```python
from build123d import *

# Parameters (mm, degrees)
SKETCH1_W           = 22
SKETCH1_H           = 22
BOSS_EXTRUDE1_DEPTH = 63.5
CUT_EXTRUDE1_DEPTH  = 71.712445864
SKETCH3_W           = 3
SKETCH3_H           = 7
CUT_EXTRUDE2_DEPTH  = 71.712445864
BOSS_EXTRUDE2_REACH = 68.259
SKETCH4_W           = 7
SKETCH4_H           = 2
FILLET1_R           = 2
CHAMFER1_SIZE       = 3


with BuildPart() as part:
    # Sketch1 → Boss-Extrude1 (new body)
    with BuildSketch(Plane.XY):
        with Locations((11, 11)):
            Rectangle(SKETCH1_W, SKETCH1_H)
    extrude(amount=-BOSS_EXTRUDE1_DEPTH)

    # Sketch2 → Cut-Extrude1 (cut, through all)
    with BuildSketch(Plane(origin=(22, 0, 0), x_dir=(0, 0, -1), z_dir=(1, 0, 0))):
        Polygon((5, 22), (5, 15), (22.833333333, 15), (22.833333333, 17), (40.666666667, 17), (40.666666667, 15), (58.5, 15), (58.5, 22), align=None)
        Polygon((22.833333333, 7), (22.833333333, 5), (40.666666667, 5), (40.666666667, 7), (58.5, 7), (58.5, 0), (5, 0), (5, 7), align=None)
    extrude(amount=-CUT_EXTRUDE1_DEPTH, mode=Mode.SUBTRACT)

    # Sketch3 → Cut-Extrude2 (cut, through all)
    with BuildSketch(Plane.XY):
        with Locations((11, 11)):
            Rectangle(SKETCH3_W, SKETCH3_H)
    extrude(amount=-CUT_EXTRUDE2_DEPTH, mode=Mode.SUBTRACT)

    # Boss-Extrude2: up to this face of the body (flat: up to its plane)
    boss_extrude2_end = Plane(part.part.faces().sort_by_distance((11, 18.5, -58.5))[0])
    # Sketch4 → Boss-Extrude2 (add, up to the picked face)
    with BuildSketch(Plane(origin=(0, 0, -5), x_dir=(-1, 0, 0), z_dir=(0, 0, -1)), mode=Mode.PRIVATE) as boss_extrude2_sk1:
        with Locations((-11, 16)):
            Rectangle(SKETCH4_W, SKETCH4_H)
    boss_extrude2_tool1 = split(extrude(boss_extrude2_sk1.sketch, amount=BOSS_EXTRUDE2_REACH, mode=Mode.PRIVATE), bisect_by=boss_extrude2_end, keep=Keep.BOTH, mode=Mode.PRIVATE)
    boss_extrude2 = boss_extrude2_tool1.solids().sort_by(Axis((11, 16, -5), (0, 0, -1)))[0]
    add(boss_extrude2)

    # Mirror1: Boss-Extrude2 across plane
    add(boss_extrude2.mirror(Plane.ZX.offset(11)))

    # Fillet1
    fillet1_edges = [part.edges().sort_by_distance(p)[0] for p in [
        (7.5, 16, -40.666666667),
        (7.5, 16, -22.833333333),
        (7.5, 16, -5),
        (14.5, 16, -40.666666667),
        (14.5, 16, -22.833333333),
        (14.5, 16, -5),
        (7.5, 16, -58.5),
        (14.5, 16, -58.5),
        (14.5, 6, -58.5),
        (7.5, 6, -58.5),
        (7.5, 6, -5),
        (14.5, 6, -5),
        (14.5, 6, -22.833333333),
        (14.5, 6, -40.666666667),
        (7.5, 6, -22.833333333),
        (7.5, 6, -40.666666667),
    ]]
    fillet(fillet1_edges, radius=FILLET1_R)

    # Chamfer1
    chamfer1_edges = [part.edges().sort_by_distance(p)[0] for p in [
        (0, 0, -2.5),
        (22, 0, -2.5),
        (22, 22, -2.5),
        (0, 22, -2.5),
        (0, 22, -61),
        (22, 22, -61),
        (22, 0, -61),
        (0, 0, -61),
    ]]
    chamfer(chamfer1_edges, length=CHAMFER1_SIZE)


solid = part.part
```
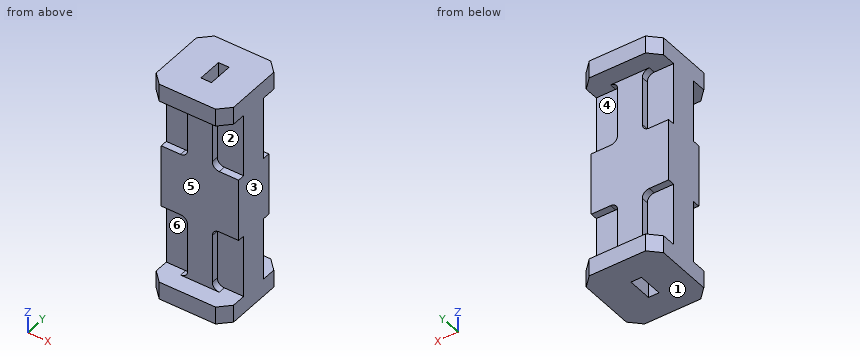
Here's how the part is built. I have some questions about the finished solid (model axes, mm). Face numbers are marked on the shaded views. A direction names the side the tool comes from. Round coordinates to 2 decimals unless told otherwise and drop trailing zeros. Order: outer loops, then holes, each group sorted by start corner. A loop starts at its lowest first (then second) coordinate and runs counter-clockwise, first axis right, second up. Notation, with made-up numbers: M 20.25,-21 L 41.25,-21 A17 ccw 41.25,-12 Z; hole C 41,32.5 d11. An arc over 180 degrees is marked long. Answer in a Markdown table with one row per item.
Item 1: Thinking about a two-plate mould opening in Z: for the marked faces 1, 2 and 3, which applies, +Z half, -Z half, draft (parallel to the pull), parting line (faces both ways), or undercut?
A:
| item | result |
|---|---|
| face 1 | -Z half |
| face 2 | undercut |
| face 3 | draft |
Item 2: I'm going to push flat-ended pins straight in: pin 1 (0.6 mm diameter, centred on y = 16.5, z = -12.5, fed in from -X); pin 2 (6 mm diameter, centred on x = 11.5, z = -33, fed in from +Y); pin 3 (2 mm diameter, centred on x = 5, z = -46.5, fed in from -Y). Where does each tip first touch, or does it pass through?
A:
| item | result |
|---|---|
| pin 1 | stops at x = 7.5 |
| pin 2 | stops at y = 17 |
| pin 3 | stops at y = 7 |
Item 3: Imagine slicing it at C-C, the plane z = -10. Write out the boundary of the cut face in (x, y).
A:
| item | result |
|---|---|
| outline | M 0,7 L 7.5,7 L 7.5,5 L 14.5,5 L 14.5,7 L 22,7 L 22,15 L 14.5,15 L 14.5,17 L 7.5,17 L 7.5,15 L 0,15 Z; hole M 9.5,7.5 L 12.5,7.5 L 12.5,14.5 L 9.5,14.5 Z |
Item 4: Imagine slicing it at D-D, the plane x = 4.75. Write out the boundary of the cut face in (y, z), and give its area (3 significant figures).
A:
| item | result |
|---|---|
| outline | M 0,-63.5 L 22,-63.5 L 22,-58.5 L 15,-58.5 L 15,-40.67 L 17,-40.67 L 17,-22.83 L 15,-22.83 L 15,-5 L 22,-5 L 22,0 L 0,0 L 0,-5 L 7,-5 L 7,-22.83 L 5,-22.83 L 5,-40.67 L 7,-40.67 L 7,-58.5 L 0,-58.5 Z |
| area | 719 mm2 |
Item 5: Imagine slicing it at B-B, the plane y = 11. Write out the boundary of the cut face in (x, z).
A:
| item | result |
|---|---|
| outline | M 0,-63.5 L 9.5,-63.5 L 9.5,0 L 0,0 Z; M 12.5,-63.5 L 22,-63.5 L 22,0 L 12.5,0 Z |
Item 6: Imagine slicing it at A-A, the plane x = 10.5. Write out the boundary of the cut face in (y, z).
A:
| item | result |
|---|---|
| outline | M 0,-63.5 L 7.5,-63.5 L 7.5,0 L 0,0 L 0,-5 L 5,-5 L 5,-58.5 L 0,-58.5 Z; M 14.5,-63.5 L 22,-63.5 L 22,-58.5 L 17,-58.5 L 17,-5 L 22,-5 L 22,0 L 14.5,0 Z |
Item 7: If I drill on L1, parallel to Z at x = 1.75, y = 17.25; L2, parallel to X at y = 9, z = -2.5; L3, parallel to Z at x = 7, y = 16.25, over which ranges is the centre line in solid material (lowest first)? Write a range as from..to.
A:
| item | result |
|---|---|
| L1 | z = -63.5..-58.5, -5..0 |
| L2 | x = 0..9.5, 12.5..22 |
| L3 | z = -63.5..-57.82, -41.34..-22.16, -5.68..0 |
Item 8: For the marked faces 4, 5 and 6, which set-ups out of +Z, -Z, +X, -X, +Y, -Y let a thin tool reach every point of the face, with its end or its side?
A:
| item | result |
|---|---|
| face 4 | +X, +Y |
| face 5 | +X, -X, -Y |
| face 6 | -X, -Y |
